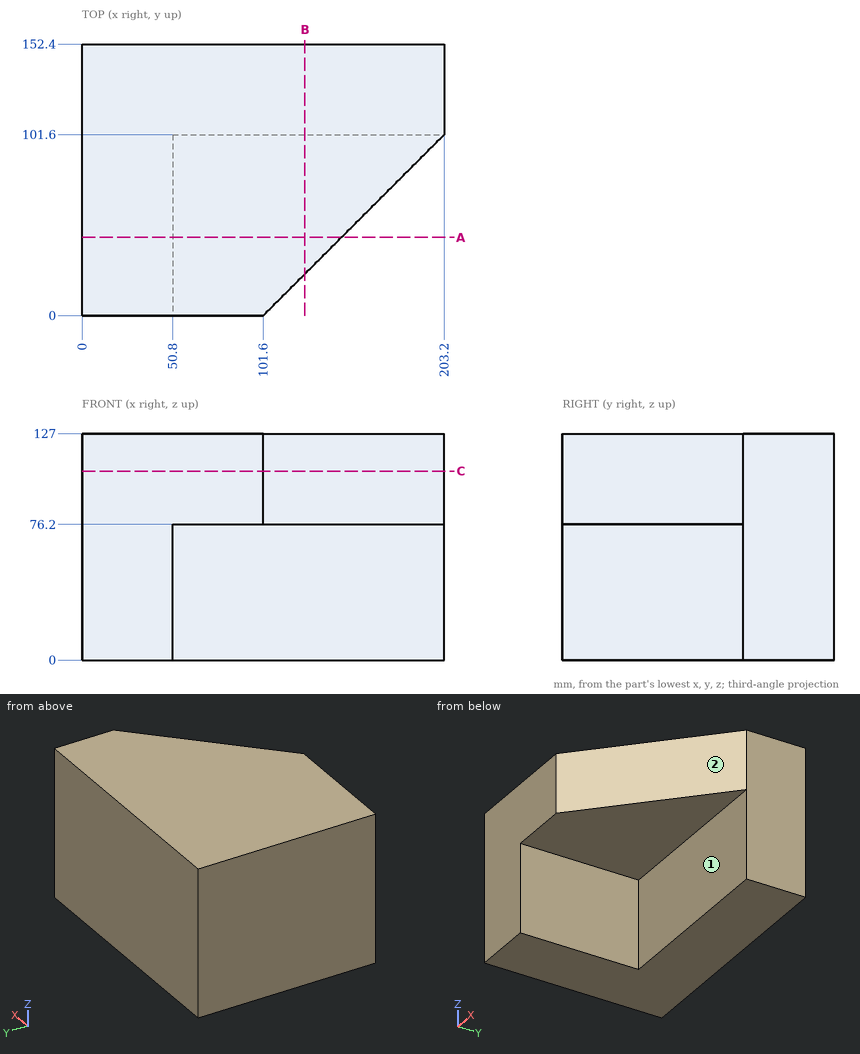
Source: three-view drawing plus pictorial views. Frame: mm from the lowest corner of the part. A direction names the side the tool comes from. Give positions to 0.01 mm unless a question says otherwise; leave off trailing zeros. Order: outer loops, then holes, each group sorted by start corner. A loop starts at its lowest first (then second) coordinate and runs counter-clockwise, first axis right, second up. Notation, with made-up numbers: (71.5, 33) -> (97.5, 33) arc R25 cw to (97.5, 72) -> close; hole circle Ø11 at (12.5, 13). An arc over 180 degrees is marked (long way). Write each question's results on one line, items separated by ' | '. Start each with the question number.
Item 1: Cut plane C-C on z = 106. Return the cut outline in (x, y), then the cut area to 3 significant figures.
Item 2: Cut plane A-A on y = 44. Return the cut outline in (x, z), then the cut area to 3 significant figures.
Item 3: Contact query for flat-ended pins moving along their axis: P1, Ø23, axis at x = 100, z = 49.5, coming from the -Y side; P2, Ø6, axis at x = 167.5, y = 86, coming from the -Z side; P3, Ø6, axis at y = 63.5, z = 30, coming from the +X side. Output: stop coordinate, or through.
Item 4: Set-up query: the marked faces 1 and 2. Return all of +Z, -Z, +X, -X, +Y, -Y with unobstructed straight access to the full face (end or side cutting, diameter ignored); none if empty.
Item 5: Line query: line 1 (Z direction, x = 59, y = 43); line 2 (Y direction, x = 153, z = 57.5); line 3 (X direction, y = 33, z = 19). Output: solid intervals per line, ascending.
Item 6: Cut plane B-B on x = 125. Return the cut outline in (y, z), then the cut area to 3 significant figures.
Established:
1) outline: (0, 0) -> (101.6, 0) -> (203.2, 101.6) -> (203.2, 152.4) -> (0, 152.4) -> close | area: 25,800 mm^2
2) outline: (0, 0) -> (50.8, 0) -> (50.8, 76.2) -> (145.6, 76.2) -> (145.6, 127) -> (0, 127) -> close | area: 11,300 mm^2
3) P1: y = 101.6 | P2: z = 76.2 | P3: x = 50.8
4) face 1: -Z, +X, -Y | face 2: +Z, -Z, +X, -Y
5) line 1: 76.2 to 127 | line 2: 101.6 to 152.4 | line 3: 0 to 50.8
6) outline: (23.4, 76.2) -> (101.6, 76.2) -> (101.6, 0) -> (152.4, 0) -> (152.4, 127) -> (23.4, 127) -> close | area: 10,400 mm^2
